Design review of the part built by this model. Coordinates are the model's own, in mm. Face numbers are marked on the shaded views. A direction names the side the tool comes from. Coordinates: 2 decimals unless noted, no trailing zeros. Loops run counter-clockwise (first coordinate to the right, second up) from the corner with the lowest first, then second, coordinate; pieces in that order, holes last. Notation, with made-up numbers: M -35.5,66.5 L -21.5,66.5 A32 cw -21.5,95.5 Z; hole C 18.25,-28 d11. An arc over 180 degrees is marked long. Answer as a JSON object with one key per item and string values. Group by question number.
1. Insertion check: pin 1 (1 mm diameter, centred on x = 35, y = 13.5, fed in from +Z); pin 2 (3.5 mm diameter, centred on x = -56, y = 23, fed in from +Z); pin 3 (6 mm diameter, centred on x = -53, y = -28, fed in from +Z). Each pin has a flat end and moves straight along its axis. Give the tip position at first contact, or say it passes through.
2. Draft analysis for pull direction Y (two halves, no side actions). For the marked faces 1, 2 and 3, state which applies: +Y half, -Y half, draft (parallel to the pull), parting line (faces both ways), or undercut.
3. Consider section B-B (x = 15.5). State the section outline as (y, z) points, then the cut area to 3 significant figures.
4. Consider section A-A (y = -9). State the section outline as (x, z) points, then the cut area to 3 significant figures.
5. To check wall thickness, follow probe 1 along Y at (x, z) = (60.5, 24.25); probe 2 along Y at (x, z) = (61, 17); probe 3 along Y at (x, z) = (79, 14). State the ranges of each line that lie inside material, in increasing order.
6. Machinability: for the marked faces 4 and 5, which of the approach directions +Z, -Z, +X, -X, +Y, -Y give a long, thin tool a straight path to every point of the face, cutting with its end or side? Answer none if there is none.
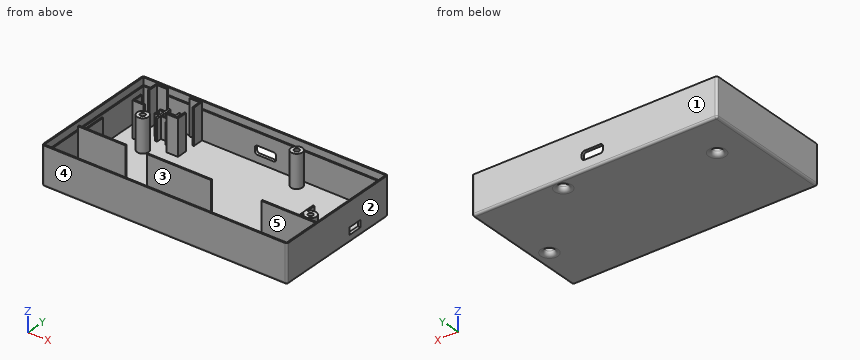
from build123d import *

# Parameters (mm, degrees)
SKETCH_1_W          = 172
SKETCH_1_H          = 92
EXTRUDE_1_DEPTH     = 2
SKETCH_2_W          = 172
SKETCH_2_H          = 92
SKETCH_2_W_2        = 168
SKETCH_2_H_2        = 88
EXTRUDE_2_DEPTH     = 25
EXTRUDE_3_DEPTH     = 25
SKETCH_4_W          = 5.927900585
SKETCH_4_H          = 3.296231716
EXTRUDE_4_DEPTH     = 15
SKETCH_5_R          = 4
EXTRUDE_5_DEPTH     = 23
SKETCH_6_R          = 1.75
CUT_EXTRUDE_1_DEPTH = 30
SKETCH_7_R          = 3
CUT_EXTRUDE_2_DEPTH = 22
SKETCH_8_R          = 4
EXTRUDE_6_DEPTH     = 23
SKETCH_9_R          = 1.75
CUT_EXTRUDE_3_DEPTH = 30
SKETCH_10_R         = 1.75
CUT_EXTRUDE_4_DEPTH = 30
SKETCH_11_R         = 3
CUT_EXTRUDE_5_DEPTH = 22
SKETCH_12_W         = 44.771170363
SKETCH_12_H         = 1
EXTRUDE_7_DEPTH     = 23
SKETCH_13_W         = 15
SKETCH_13_H         = 6
CUT_EXTRUDE_6_DEPTH = 23
FILLET_1_R          = 2
FILLET_2_R          = 3
SKETCH_14_W         = 5
SKETCH_14_H         = 10
CUT_EXTRUDE_7_DEPTH = 23
SKETCH_15_W         = 170
SKETCH_15_H         = 90
CUT_EXTRUDE_8_DEPTH = 5
FILLET_3_R          = 1.5


with BuildPart() as part:
    # 草图1 → 凸台-拉伸1 (new body)
    with BuildSketch(Plane.XY):
        with Locations((3.714694656, -11.181774809)):
            Rectangle(SKETCH_1_W, SKETCH_1_H)
    extrude(amount=EXTRUDE_1_DEPTH)

    # 草图2 → 凸台-拉伸2 (add)
    with BuildSketch(Plane.XY.offset(2)):
        with Locations((3.714694656, -11.181774809)):
            Rectangle(SKETCH_2_W, SKETCH_2_H)
        with Locations((3.714694656, -11.181774809)):
            Rectangle(SKETCH_2_W_2, SKETCH_2_H_2, mode=Mode.SUBTRACT)
    extrude(amount=EXTRUDE_2_DEPTH)

    # 草图3 → 凸台-拉伸3 (add)
    with BuildSketch(Plane.XY.offset(2)):
        Polygon((-71.285305344, 32.818225191), (-63.285305344, 32.818225191), (-63.285305344, 31.818225191), (-70.285305344, 31.818225191), (-70.285305344, 25.318225191), (-71.285305344, 25.318225191), align=None)
        Polygon((-71.285305344, 10.818225191), (-63.285305344, 10.818225191), (-63.285305344, 11.818225191), (-70.285305344, 11.818225191), (-70.285305344, 18.318225191), (-71.285305344, 18.318225191), align=None)
        Polygon((-39.285305344, 32.818225191), (-39.285305344, 25.318225191), (-40.285305344, 25.318225191), (-40.285305344, 31.818225191), (-47.285305344, 31.818225191), (-47.285305344, 32.818225191), align=None)
        Polygon((-40.285305344, 18.318225191), (-39.285305344, 18.318225191), (-39.285305344, 10.818225191), (-47.285305344, 10.818225191), (-47.285305344, 11.818225191), (-40.285305344, 11.818225191), align=None)
    extrude(amount=EXTRUDE_3_DEPTH)

    # 草图4 → 凸台-拉伸4 (add)
    with BuildSketch(Plane.XY.offset(2)):
        Polygon((-59.649980097, 24.438275263), (-59.649980097, 21.142043547), (-62.919629299, 21.142043547), (-62.919629299, 19.972412939), (-59.649980097, 19.972412939), (-59.649980097, 16.543268654), (-58.267689377, 16.543268654), (-58.267689377, 19.972412939), (-52.339788792, 19.972412939), (-52.339788792, 16.543268654), (-50.904333045, 16.543268654), (-50.904333045, 19.972412939), (-47.608101329, 19.972412939), (-47.608101329, 21.142043547), (-50.904333045, 21.142043547), (-50.904333045, 24.438275263), (-47.608101329, 24.438275263), (-47.608101329, 25.528158331), (-50.904333045, 25.528158331), (-50.904333045, 28.85097256), (-52.339788792, 28.85097256), (-52.339788792, 25.528158331), (-58.267689377, 25.528158331), (-58.267689377, 28.85097256), (-59.649980097, 28.85097256), (-59.649980097, 25.528158331), (-62.919629299, 25.528158331), (-62.919629299, 24.438275263), align=None)
        with Locations((-55.303739085, 22.790159405)):
            Rectangle(SKETCH_4_W, SKETCH_4_H, mode=Mode.SUBTRACT)
    extrude(amount=EXTRUDE_4_DEPTH)

    # 草图5 → 凸台-拉伸5 (add)
    with BuildSketch(Plane.XY.offset(2)):
        with Locations(Location((-59.285305344, 4.818225191, 0), (0, 0, 180))):
            Circle(SKETCH_5_R)
    extrude(amount=EXTRUDE_5_DEPTH)

    # 草图6 → 切除-拉伸1 (cut)
    with BuildSketch(Plane.XY.offset(25)):
        with Locations((-59.285305344, 4.818225191)):
            Circle(SKETCH_6_R)
    extrude(amount=-CUT_EXTRUDE_1_DEPTH, mode=Mode.SUBTRACT)

    # 草图7 → 切除-拉伸2 (cut)
    with BuildSketch(Plane(origin=(0, 0, 0), x_dir=(-1, 0, 0), z_dir=(0, 0, -1))):
        with Locations((59.285305344, 4.818225191)):
            Circle(SKETCH_7_R)
    extrude(amount=-CUT_EXTRUDE_2_DEPTH, mode=Mode.SUBTRACT)

    # 草图8 → 凸台-拉伸6 (add)
    with BuildSketch(Plane.XY.offset(2)):
        with Locations(Location((31.392694656, 27.297225191, 0), (0, 0, 180))):
            Circle(SKETCH_8_R)
        with Locations(Location((79.144694656, -21.978774809, 0), (0, 0, 180))):
            Circle(SKETCH_8_R)
    extrude(amount=EXTRUDE_6_DEPTH)

    # 草图9 → 切除-拉伸3 (cut)
    with BuildSketch(Plane.XY.offset(25)):
        with Locations((31.392694656, 27.297225191)):
            Circle(SKETCH_9_R)
    extrude(amount=-CUT_EXTRUDE_3_DEPTH, mode=Mode.SUBTRACT)

    # 草图10 → 切除-拉伸4 (cut)
    with BuildSketch(Plane.XY.offset(25)):
        with Locations((79.144694656, -21.978774809)):
            Circle(SKETCH_10_R)
    extrude(amount=-CUT_EXTRUDE_4_DEPTH, mode=Mode.SUBTRACT)

    # 草图11 → 切除-拉伸5 (cut)
    with BuildSketch(Plane(origin=(0, 0, 0), x_dir=(-1, 0, 0), z_dir=(0, 0, -1))):
        with Locations((-31.392694656, 27.297225191)):
            Circle(SKETCH_11_R)
        with Locations((-79.144694656, -21.978774809)):
            Circle(SKETCH_11_R)
    extrude(amount=-CUT_EXTRUDE_5_DEPTH, mode=Mode.SUBTRACT)

    # 草图12 → 凸台-拉伸7 (add)
    with BuildSketch(Plane.XY.offset(2)):
        Polygon((87.714694656, -26.239681565), (75.367291859, -26.239681565), (75.367291859, -13.468786918), (74.367291859, -13.468786918), (74.367291859, -26.239681565), (48.560091816, -26.239681565), (48.560091816, -27.239681565), (87.714694656, -27.239681565), align=None)
        Polygon((-80.285305344, -25.958692289), (-75.644143466, -25.958692289), (-75.644143466, -11.323392388), (-74.644143466, -11.323392388), (-74.644143466, -25.958692289), (-46.929156899, -25.958692289), (-46.929156899, -26.958692289), (-80.285305344, -26.958692289), align=None)
        with Locations((-9.415382556, -26.458692289)):
            Rectangle(SKETCH_12_W, SKETCH_12_H)
    extrude(amount=EXTRUDE_7_DEPTH)

    # 草图13 → 切除-拉伸6 (cut)
    with BuildSketch(Plane(origin=(0, 34.818225191, 0), x_dir=(1, 0, 0), z_dir=(0, 1, 0))):
        with Locations((5.214694656, -10.2)):
            Rectangle(SKETCH_13_W, SKETCH_13_H)
    extrude(amount=-CUT_EXTRUDE_6_DEPTH, mode=Mode.SUBTRACT)

    # 圆角1
    fillet_1_edges = [part.edges().sort_by_distance(p)[0] for p in [
        (-2.285305344, 33.818225191, 13.2),
        (-2.285305344, 33.818225191, 7.2),
        (12.714694656, 33.818225191, 7.2),
        (12.714694656, 33.818225191, 13.2),
    ]]
    fillet(fillet_1_edges, radius=FILLET_1_R)

    # 圆角2
    fillet_2_edges = [part.edges().sort_by_distance(p)[0] for p in [
        (-56.285305344, 4.818225191, 0),
        (34.392694656, 27.297225191, 0),
        (82.144694656, -21.978774809, 0),
    ]]
    fillet(fillet_2_edges, radius=FILLET_2_R)

    # 草图14 → 切除-拉伸7 (cut)
    with BuildSketch(Plane(origin=(89.714694656, 0, 0), x_dir=(0, 0, -1), z_dir=(1, 0, 0))):
        with Locations((-7.5, 4.818225191)):
            Rectangle(SKETCH_14_W, SKETCH_14_H)
    extrude(amount=-CUT_EXTRUDE_7_DEPTH, mode=Mode.SUBTRACT)

    # 草图15 → 切除-拉伸8 (cut)
    with BuildSketch(Plane.XY.offset(27)):
        with Locations((3.714694656, -11.181774809)):
            Rectangle(SKETCH_15_W, SKETCH_15_H)
        Polygon((-80.285305344, 32.818225191), (-71.285305344, 32.818225191), (-63.285305344, 32.818225191), (-47.285305344, 32.818225191), (-39.285305344, 32.818225191), (87.714694656, 32.818225191), (87.714694656, -55.181774809), (-80.285305344, -55.181774809), align=None, mode=Mode.SUBTRACT)
    extrude(amount=-CUT_EXTRUDE_8_DEPTH, mode=Mode.SUBTRACT)

    # 圆角3
    fillet_3_edges = [part.edges().sort_by_distance(p)[0] for p in [
        (-82.285305344, -11.181774809, 0),
        (3.714694656, 34.818225191, 0),
        (89.714694656, -11.181774809, 0),
        (3.714694656, -57.181774809, 0),
        (-82.285305344, -57.181774809, 13.5),
        (-82.285305344, 34.818225191, 13.5),
        (89.714694656, 34.818225191, 13.5),
        (89.714694656, -57.181774809, 13.5),
    ]]
    fillet(fillet_3_edges, radius=FILLET_3_R)


solid = part.part
Findings below:
{
 "1": {"pin 1": "stops at z = 2", "pin 2": "stops at z = 17", "pin 3": "stops at z = 25"},
 "2": {"face 1": "+Y half", "face 2": "draft", "face 3": "undercut"},
 "3": {"outline": "M -57.18,1.5 A1.5 ccw -55.68,0 L 33.32,0 A1.5 ccw 34.82,1.5 L 34.82,27 L 33.82,27 L 33.82,22 L 32.82,22 L 32.82,2 L -55.18,2 L -55.18,22 L -56.18,22 L -56.18,27 L -57.18,27 Z", "area": "273 mm^2"},
 "4": {"outline": "M -82.29,1.5 A1.5 ccw -80.79,0 L 88.21,0 A1.5 ccw 89.71,1.5 L 89.71,27 L 88.71,27 L 88.71,22 L 87.71,22 L 87.71,2 L -80.29,2 L -80.29,22 L -81.29,22 L -81.29,27 L -82.29,27 Z", "area": "433 mm^2"},
 "5": {"probe 1": "y = -57.18 to -56.18, -27.24 to -26.24, 33.82 to 34.82", "probe 2": "y = -57.18 to -55.18, -27.24 to -26.24, 32.82 to 34.82", "probe 3": "y = -57.18 to -55.18, -27.24 to -26.24, -25.98 to -24.98, -18.98 to -17.98, 32.82 to 34.82"},
 "6": {"face 4": "+Z, -Z, +X, -X, -Y", "face 5": "+Z"}
}
